The listing builds one solid part. Answer for the finished solid, in the listing's coordinates (mm). Face numbers are marked on the shaded views. A direction names the side the tool comes from. Give positions to 0.01 mm unless a question says otherwise; leave off trailing zeros. Loops run counter-clockwise (first coordinate to the right, second up) from the corner with the lowest first, then second, coordinate; pieces in that order, holes last.
Item 1: The mould has two halves that part along Y. Classify the marked faces 3, 4 and 5: pulls with the +Y half, pulls with the -Y half, needs draft (parallel to the pull), parting line crosses it, or undercut.
Item 2: Section C-C, the plane y = 0 is taken. Give the vertices of the cut face in (x, z), and give its area (3 significant figures).
Item 3: Consider line 1 along Y through (x, z) = (-7, 26.5); line 2 along Z through (x, y) = (-10, -7); line 3 along X through (y, z) = (3.5, 6.5). Determine where each line is inside the solid, lowest interval first.
Item 4: A tool of negligible diameter and unlimited length cuts with its end or side. For the marked faces 1 and 2, from which of +Z, -Z, +X, -X, +Y, -Y can it reach the whole face along a straight path? Write none if from no direction.
Item 5: Section B-B, the plane z = 11 is taken. Give the vertices of the cut face in (x, y), and give its area (3 significant figures).
Item 6: Section D-D, the plane x = -7.5 is taken. Give the vertices of the cut face in (y, z).
Item 7: Section A-A, the plane x = -4 is taken. Give the vertices of the cut face in (y, z).
Item 8: Each of these flat-tipped pins is pushed along its axis until it touches: pin 1 Ø1 at (x, y) = (-14.5, -4) entering from +Z; pin 2 Ø1 at (y, z) = (-13, 23.5) entering from +X; pin 3 Ø4 at (y, z) = (8, 31.5) entering from +X; pin 4 Ø10 at (x, z) = (1.5, 34.5) entering from -Y. Where does it stop, or does it pass through?
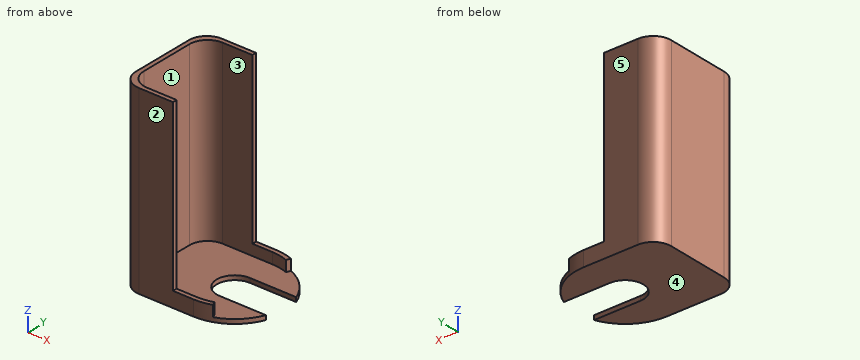
from build123d import *

# Parameters (mm, degrees)
F1_DEPTH = 1.2
F2_DEPTH = 49
F4_DEPTH = 46


# Not quite as in the source:
# - a feature names something its author has since deleted; it is built from what else it names


with BuildPart() as f1:
    # F0 (on Top) → F1 (new body)
    with BuildSketch(Plane.XY):
        with BuildLine():
            Line((-15, -13.7), (0, -13.7))
            ThreePointArc((0, -13.7), (2.378980034, -13.4918662163), (4.6856759636, -12.8737889048))
            Line((4.6856759636, -12.8737889048), (4.2752517916, -11.7461577598))
            ThreePointArc((4.2752517916, -11.7461577598), (2.1706022208, -12.3100969127), (0, -12.5))
            Line((0, -12.5), (-13.8, -12.5))
            ThreePointArc((-13.8, -12.5), (-17.3355339059, -11.0355339059), (-18.8, -7.5))
            Line((-18.8, -7.5), (-18.8, 7.5))
            ThreePointArc((-18.8, 7.5), (-17.3355339059, 11.0355339059), (-13.8, 12.5))
            Line((-13.8, 12.5), (0, 12.5))
            ThreePointArc((0, 12.5), (2.1706022208, 12.3100969127), (4.2752517916, 11.7461577598))
            Line((4.2752517916, 11.7461577598), (4.6856759636, 12.8737889048))
            ThreePointArc((4.6856759636, 12.8737889048), (2.378980034, 13.4918662163), (0, 13.7))
            Line((0, 13.7), (-15, 13.7))
            ThreePointArc((-15, 13.7), (-18.5355339059, 12.2355339059), (-20, 8.7))
            Line((-20, 8.7), (-20, -8.7))
            ThreePointArc((-20, -8.7), (-18.5355339059, -12.2355339059), (-15, -13.7))
        make_face()
        with BuildLine():
            Line((4.2752517916, -11.7461577598), (4.6856759636, -12.8737889048))
            ThreePointArc((4.6856759636, -12.8737889048), (9.5678327692, -9.8054360485), (12.75499902, -5))
            Line((12.75499902, -5), (11.4564392374, -5))
            ThreePointArc((11.4564392374, -5), (8.5585738758, -9.1104782099), (4.2752517916, -11.7461577598))
        make_face()
        with BuildLine():
            ThreePointArc((0, -12.5), (2.1706022208, -12.3100969127), (4.2752517916, -11.7461577598))
            ThreePointArc((4.2752517916, -11.7461577598), (8.5585738758, -9.1104782099), (11.4564392374, -5))
            Line((11.4564392374, -5), (0, -5))
            ThreePointArc((0, -5), (-5, 0), (0, 5))
            Line((0, 5), (11.4564392374, 5))
            ThreePointArc((11.4564392374, 5), (8.5585738758, 9.1104782099), (4.2752517916, 11.7461577598))
            ThreePointArc((4.2752517916, 11.7461577598), (2.1706022208, 12.3100969127), (0, 12.5))
            Line((0, 12.5), (-13.8, 12.5))
            ThreePointArc((-13.8, 12.5), (-17.3355339059, 11.0355339059), (-18.8, 7.5))
            Line((-18.8, 7.5), (-18.8, -7.5))
            ThreePointArc((-18.8, -7.5), (-17.3355339059, -11.0355339059), (-13.8, -12.5))
            Line((-13.8, -12.5), (0, -12.5))
        make_face()
        with BuildLine():
            ThreePointArc((4.2752517916, 11.7461577598), (8.5585738758, 9.1104782099), (11.4564392374, 5))
            Line((11.4564392374, 5), (12.75499902, 5))
            ThreePointArc((12.75499902, 5), (9.5678327692, 9.8054360485), (4.6856759636, 12.8737889048))
            Line((4.6856759636, 12.8737889048), (4.2752517916, 11.7461577598))
        make_face()
    extrude(amount=-F1_DEPTH)

    # F0 (on Top) → F2 (join)
    with BuildSketch(Plane.XY):
        with BuildLine():
            Line((-15, -13.7), (0, -13.7))
            ThreePointArc((0, -13.7), (2.378980034, -13.4918662163), (4.6856759636, -12.8737889048))
            Line((4.6856759636, -12.8737889048), (4.2752517916, -11.7461577598))
            ThreePointArc((4.2752517916, -11.7461577598), (2.1706022208, -12.3100969127), (0, -12.5))
            Line((0, -12.5), (-13.8, -12.5))
            ThreePointArc((-13.8, -12.5), (-17.3355339059, -11.0355339059), (-18.8, -7.5))
            Line((-18.8, -7.5), (-18.8, 7.5))
            ThreePointArc((-18.8, 7.5), (-17.3355339059, 11.0355339059), (-13.8, 12.5))
            Line((-13.8, 12.5), (0, 12.5))
            ThreePointArc((0, 12.5), (2.1706022208, 12.3100969127), (4.2752517916, 11.7461577598))
            Line((4.2752517916, 11.7461577598), (4.6856759636, 12.8737889048))
            ThreePointArc((4.6856759636, 12.8737889048), (2.378980034, 13.4918662163), (0, 13.7))
            Line((0, 13.7), (-15, 13.7))
            ThreePointArc((-15, 13.7), (-18.5355339059, 12.2355339059), (-20, 8.7))
            Line((-20, 8.7), (-20, -8.7))
            ThreePointArc((-20, -8.7), (-18.5355339059, -12.2355339059), (-15, -13.7))
        make_face()
    extrude(amount=F2_DEPTH)

    # F3 (on face) → F4 (cut)
    with BuildSketch(Plane.XY.offset(49)):
        with BuildLine():
            ThreePointArc((-5.6071383076, 12.5), (-2.8670542374, 13.3966413701), (0, 13.7))
            Line((0, 13.7), (-5.6071383076, 13.7))
            Line((-5.6071383076, 13.7), (-5.6071383076, 12.5))
        make_face()
        with BuildLine():
            Line((4.2752517916, 11.7461577598), (4.6856759636, 12.8737889048))
            ThreePointArc((4.6856759636, 12.8737889048), (2.378980034, 13.4918662163), (0, 13.7))
            ThreePointArc((0, 13.7), (-2.8670542374, 13.3966413701), (-5.6071383076, 12.5))
            Line((-5.6071383076, 12.5), (0, 12.5))
            ThreePointArc((0, 12.5), (2.1706022208, 12.3100969127), (4.2752517916, 11.7461577598))
        make_face()
        with BuildLine():
            ThreePointArc((0, -13.7), (2.378980034, -13.4918662163), (4.6856759636, -12.8737889048))
            Line((4.6856759636, -12.8737889048), (4.2752517916, -11.7461577598))
            ThreePointArc((4.2752517916, -11.7461577598), (2.1706022208, -12.3100969127), (0, -12.5))
            Line((0, -12.5), (-5.6071383076, -12.5))
            ThreePointArc((-5.6071383076, -12.5), (-2.8670542374, -13.3966413701), (0, -13.7))
        make_face()
        with BuildLine():
            Line((-5.6071383076, -13.7), (0, -13.7))
            ThreePointArc((0, -13.7), (-2.8670542374, -13.3966413701), (-5.6071383076, -12.5))
            Line((-5.6071383076, -12.5), (-5.6071383076, -13.7))
        make_face()
    extrude(amount=-F4_DEPTH, mode=Mode.SUBTRACT)


solid = f1.part
Worked answers:
1. face 3: undercut
1. face 4: needs draft
1. face 5: pulls with the +Y half
2. outline: (-20, -1.2) - (-5, -1.2) - (-5, 0) - (-18.8, 0) - (-18.8, 49) - (-20, 49) - close
2. area: 76.8 mm2
3. line 1: y = -13.7 to -12.5, 12.5 to 13.7
3. line 2: z = -1.2 to 0
3. line 3: x = -20 to -18.8
4. face 1: +Z, +X
4. face 2: +Z, -Z, +X, -X, -Y
5. outline: (-20, -8.7) arc R5 ccw to (-15, -13.7) - (-5.61, -13.7) - (-5.61, -12.5) - (-13.8, -12.5) arc R5 cw to (-18.8, -7.5) - (-18.8, 7.5) arc R5 cw to (-13.8, 12.5) - (-5.61, 12.5) - (-5.61, 13.7) - (-15, 13.7) arc R5 ccw to (-20, 8.7) - close
5. area: 64.5 mm2
6. outline: (-13.7, -1.2) - (13.7, -1.2) - (13.7, 49) - (12.5, 49) - (12.5, 0) - (-12.5, 0) - (-12.5, 49) - (-13.7, 49) - close
7. outline: (-13.7, -1.2) - (-3, -1.2) - (-3, 0) - (-12.5, 0) - (-12.5, 3) - (-13.7, 3) - close; (3, -1.2) - (13.7, -1.2) - (13.7, 3) - (12.5, 3) - (12.5, 0) - (3, 0) - close
8. pin 1: stops at z = 0
8. pin 2: stops at x = -5.61
8. pin 3: stops at x = -18.13
8. pin 4: passes through
